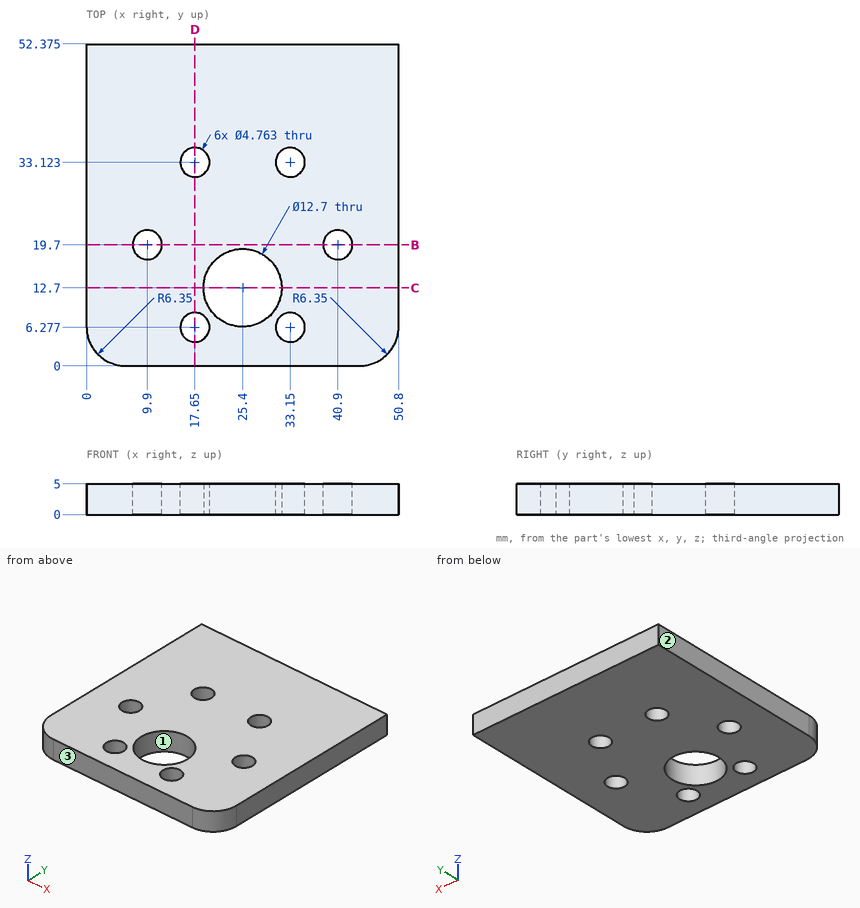
Can you work these out from the drawing? Everything is in mm from the part's minimum corner. Coordinates: 2 decimals unless noted, no trailing zeros. Write each loop counter-clockwise with the first axis right and the second up, starting at its lowest first coordinate (ties: lowest second). Pieces come first, ordered by that corner, then holes. Notation, with made-up numbers: (-32.75, 54) - (-22.75, 54) arc R24 cw to (-22.75, 86) - close; hole circle Ø11 at (-25.5, 13). An arc over 180 degrees is marked (long way). One line per item, written item: value.
1) Suppose I cut it at D-D on x = 17.65. Write out the boundary of the cut face in (y, z) (1 decimal), and give its area (3 significant figures).
Model answer:
outline: (0, 0) - (3.9, 0) - (3.9, 5) - (0, 5) - close; (8.7, 0) - (30.7, 0) - (30.7, 5) - (8.7, 5) - close; (35.5, 0) - (52.4, 0) - (52.4, 5) - (35.5, 5) - close
area: 214 mm²
2) Suppose I cut it at B-B on y = 19.7. Write out the boundary of the cut face in (x, z), and give its area (3 significant figures).
Model answer:
outline: (0, 0) - (7.52, 0) - (7.52, 5) - (0, 5) - close; (12.28, 0) - (38.52, 0) - (38.52, 5) - (12.28, 5) - close; (43.28, 0) - (50.8, 0) - (50.8, 5) - (43.28, 5) - close
area: 206 mm²
3) Suppose I cut it at C-C on y = 12.7. Write out the boundary of the cut face in (x, z).
Model answer:
outline: (0, 0) - (19.05, 0) - (19.05, 5) - (0, 5) - close; (31.75, 0) - (50.8, 0) - (50.8, 5) - (31.75, 5) - close
4) I need wall thicknesses on line 1 along Y through (x, z) = (17.65, 3.6) (1 decimal); line 2 along X through (y, z) = (34, 2.8) (1 decimal); line 3 along Y through (x, z) = (32, 0.3) (1 decimal). Which ranges of each line are inside material? Lowest first, please.
Model answer:
line 1: y = 0 to 3.9, 8.7 to 30.7, 35.5 to 52.4
line 2: x = 0 to 15.4, 19.9 to 30.9, 35.4 to 50.8
line 3: y = 0 to 4.2, 8.4 to 31, 35.2 to 52.4
5) We'd pull the mould along X, two halves only. Please class the marked faces 1, 2 and 3: pulls with the +X half, pulls with the -X half, needs draft (parallel to the pull), parting line crosses it, or undercut.
Model answer:
face 1: undercut
face 2: pulls with the -X half
face 3: needs draft
